Source: CAD feature listing. Evaluate the final solid. Frame: model axes, mm. A direction names the side the tool comes from. Give positions to 0.01 mm unless a question says otherwise; leave off trailing zeros. Order: outer loops, then holes, each group sorted by start corner. A loop starts at its lowest first (then second) coordinate and runs counter-clockwise, first axis right, second up.
from build123d import *

# Parameters (mm, degrees)
DODANIE_WYCI_GNI_CIE1_DEPTH = 1.9
DODANIE_WYCI_GNI_CIE3_DEPTH = 12.4
ESQUISSE4_R                 = 2.2
BOSS_EXTRU_2_DEPTH          = 2
ESQUISSE5_R                 = 1.1
ENL_V_MAT_EXTRU_2_DEPTH     = 29.971882921
ENL_V_MAT_EXTRU_4_REACH     = 38.806
ESQUISSE6_R                 = 1.1
ENL_V_START                 = -2.2
ESQUISSE7_R                 = 1.6
ESQUISSE7_R_2               = 1.1
ENL_V_MAT_EXTRU_5_DEPTH     = 2.2


with BuildPart() as part:
    # Szkic1 → Dodanie-wyciągnięcie1 (new body)
    with BuildSketch(Plane.XY):
        with BuildLine():
            Line((-12.9, 20), (12.9, 20))
            ThreePointArc((12.9, 20), (15.728427125, 18.828427125), (16.9, 16))
            Line((16.9, 16), (16.9, -16))
            ThreePointArc((16.9, -16), (15.728427125, -18.828427125), (12.9, -20))
            Line((12.9, -20), (-12.9, -20))
            ThreePointArc((-12.9, -20), (-15.728427125, -18.828427125), (-16.9, -16))
            Line((-16.9, -16), (-16.9, 16))
            ThreePointArc((-16.9, 16), (-15.728427125, 18.828427125), (-12.9, 20))
        make_face()
    extrude(amount=DODANIE_WYCI_GNI_CIE1_DEPTH)

    # Szkic3 → Dodanie-wyciągnięcie3 (add)
    with BuildSketch(Plane(origin=(0, 0, 0), x_dir=(-1, 0, 0), z_dir=(0, 0, -1))):
        Polygon((-9.4, -16.5), (-9.4, -11.5), (-11.4, -11.5), (-11.4, -18.5), (-2, -18.5), (-2, -11.5), (-6.5, -11.5), (-6.5, -16.5), align=None)
        Polygon((-9.4, 11.5), (-11.4, 11.5), (-11.4, 18.5), (-2, 18.5), (-2, 11.5), (-6.5, 11.5), (-6.5, 16.5), (-9.4, 16.5), align=None)
    extrude(amount=DODANIE_WYCI_GNI_CIE3_DEPTH)

    # Esquisse4 → Boss.-Extru.2 (add)
    with BuildSketch(Plane.ZY.offset(16.9)):
        with BuildLine():
            Line((-3.579120726, 8.391358342), (0, 5.442162864))
            Line((0, 5.442162864), (0, -5.442162864))
            Line((0, -5.442162864), (-8.920879274, 1.908641658))
            ThreePointArc((-8.920879274, 1.908641658), (-9.491358342, 7.820879274), (-3.579120726, 8.391358342))
        make_face()
        with Locations(Location((-6.25, 5.15, 0), (0, 0, 270))):
            Circle(ESQUISSE4_R, mode=Mode.SUBTRACT)
    extrude(amount=-BOSS_EXTRU_2_DEPTH)

    # Esquisse5 → Enlèv. mat.-Extru.2 (cut, through all)
    with BuildSketch(Plane(origin=(0, 0, 0), x_dir=(-1, 0, 0), z_dir=(0, 0, -1))):
        with Locations((6, 16)):
            Circle(ESQUISSE5_R)
        with Locations((6, -16)):
            Circle(ESQUISSE5_R)
    extrude(amount=-ENL_V_MAT_EXTRU_2_DEPTH, mode=Mode.SUBTRACT)

    # Enlèv. mat.-Extru.4: up to this face of the body (flat: up to its plane)
    enl_v_mat_extru_4_end = Plane(part.part.faces().sort_by_distance((2, 15, -6.2))[0])
    # Esquisse6 → Enlèv. mat.-Extru.4 (cut, up to the picked face)
    with BuildSketch(Plane(origin=(11.4, 0, 0), x_dir=(0, 0, -1), z_dir=(1, 0, 0)), mode=Mode.PRIVATE) as enl_v_mat_extru_4_sk1:
        with Locations((6.2, 13.9)):
            Circle(ESQUISSE6_R)
    enl_v_mat_extru_4_tool1 = split(extrude(enl_v_mat_extru_4_sk1.sketch, amount=-ENL_V_MAT_EXTRU_4_REACH, mode=Mode.PRIVATE), bisect_by=enl_v_mat_extru_4_end, keep=Keep.BOTH, mode=Mode.PRIVATE)
    # Esquisse6 → Enlèv. mat.-Extru.4 (cut, up to the picked face)
    with BuildSketch(Plane(origin=(11.4, 0, 0), x_dir=(0, 0, -1), z_dir=(1, 0, 0)), mode=Mode.PRIVATE) as enl_v_mat_extru_4_sk2:
        with Locations((6.2, -13.9)):
            Circle(ESQUISSE6_R)
    enl_v_mat_extru_4_tool2 = split(extrude(enl_v_mat_extru_4_sk2.sketch, amount=-ENL_V_MAT_EXTRU_4_REACH, mode=Mode.PRIVATE), bisect_by=enl_v_mat_extru_4_end, keep=Keep.BOTH, mode=Mode.PRIVATE)
    add(enl_v_mat_extru_4_tool1.solids().sort_by(Axis((11.4, 13.9, -6.2), (-1, 0, 0)))[0], mode=Mode.SUBTRACT)
    add(enl_v_mat_extru_4_tool2.solids().sort_by(Axis((11.4, -13.9, -6.2), (-1, 0, 0)))[0], mode=Mode.SUBTRACT)

    # Esquisse7 → Enlèv. mat.-Extru.5 (cut)
    # profile 1 of 4: a face of its own
    with BuildSketch(Plane.ZY.offset(-2).offset(ENL_V_START)):
        with Locations(Location((-6.2, 13.9, 0), (0, 0, 270))):
            Circle(ESQUISSE7_R)
        with Locations(Location((-6.2, 13.9, 0), (0, 0, 180))):
            Circle(ESQUISSE7_R_2, mode=Mode.SUBTRACT)
    # profile 2 of 4: a face of its own
    with BuildSketch(Plane.ZY.offset(-2).offset(ENL_V_START)):
        with Locations(Location((-6.2, 13.9, 0), (0, 0, 180))):
            Circle(ESQUISSE7_R_2)
    # profile 3 of 4: a face of its own
    with BuildSketch(Plane.ZY.offset(-2).offset(ENL_V_START)):
        with Locations(Location((-6.2, -13.9, 0), (0, 0, 270))):
            Circle(ESQUISSE7_R)
        with Locations(Location((-6.2, -13.9, 0), (0, 0, 270))):
            Circle(ESQUISSE7_R_2, mode=Mode.SUBTRACT)
    # profile 4 of 4: a face of its own
    with BuildSketch(Plane.ZY.offset(-2).offset(ENL_V_START)):
        with Locations(Location((-6.2, -13.9, 0), (0, 0, 270))):
            Circle(ESQUISSE7_R_2)
    extrude(amount=ENL_V_MAT_EXTRU_5_DEPTH, mode=Mode.SUBTRACT)


solid = part.part
1) First-contact query: pin 1 Ø4 at (x, y) = (5.5, -7.5) entering from -Z; pin 2 Ø5.5 at (y, z) = (13.5, -7) entering from +X; pin 3 Ø2.5 at (y, z) = (-13.9, -6.2) entering from -X; pin 4 Ø2 at (y, z) = (-13.9, -6.2) entering from -X. Flat tips, straight axial feed; report the tip coordinate or a pass-through.
Checks:
pin 1: stops at z = 0
pin 2: stops at x = 11.4
pin 3: stops at x = 4.2
pin 4: passes through
2) Section query A-A on x = -6. Output: boundary loops of the cut face in (y, z), and give its area (3 significant figures).
Checks:
outline: (-20, 0) - (-17.1, 0) - (-17.1, 1.9) - (-20, 1.9) - close; (-14.9, 0) - (14.9, 0) - (14.9, 1.9) - (-14.9, 1.9) - close; (17.1, 0) - (20, 0) - (20, 1.9) - (17.1, 1.9) - close
area: 67.6 mm2
3) Ray query, L1, parallel to Y at x = -6, z = 0.9; L2, parallel to X at y = 13, z = -4; L3, parallel to Y at x = 10.1, z = -6.2. Return the intervals inside material, ascending.
Checks:
L1: y = -20 to -17.1, -14.9 to 14.9, 17.1 to 20
L2: x = 2 to 6.5, 9.4 to 11.4
L3: y = -18.5 to -15, -12.8 to -11.5, 11.5 to 12.8, 15 to 18.5
4) Section query D-D on x = 10. Output: boundary loops of the cut face in (y, z).
Checks:
outline: (-20, 0) - (-18.5, 0) - (-18.5, -12.4) - (-11.5, -12.4) - (-11.5, 0) - (11.5, 0) - (11.5, -12.4) - (18.5, -12.4) - (18.5, 0) - (20, 0) - (20, 1.9) - (-20, 1.9) - close; hole circle Ø2.2 at (-13.9, -6.2); hole circle Ø2.2 at (13.9, -6.2)
5) Section query B-B on z = -1. Output: boundary loops of the cut face in (x, y), and give its area (3 significant figures).
Checks:
outline: (-16.9, -4.62) - (-14.9, -4.62) - (-14.9, 6.27) - (-16.9, 6.27) - close; (2, -18.5) - (11.4, -18.5) - (11.4, -11.5) - (9.4, -11.5) - (9.4, -16.5) - (6.5, -16.5) - (6.5, -11.5) - (2, -11.5) - close; (2, 11.5) - (6.5, 11.5) - (6.5, 16.5) - (9.4, 16.5) - (9.4, 11.5) - (11.4, 11.5) - (11.4, 18.5) - (2, 18.5) - close
area: 124 mm2
6) Pull-direction query (X, two-part tool) for faces 1 (the face through (15.759, -18.797, 0.937)), 2 (the face through (8, 16.5, -6)), 3 (the face through (2, 16, -6)); classes: +X half, -X half, draft (parallel to the pull), parting line (faces both ways), or undercut.
Checks:
face 1: +X half
face 2: undercut
face 3: -X half
7) Reachability of faces 4 (the face through (4.2, 15, -7)), 5 (the face through (6.5, 14, -4.7)), 6 (the face through (-14.9, 4, -4)) from +Z, -Z, +X, -X, +Y, -Y: full face, straight path, thin tool, end or side. Return the list, or none.
Checks:
face 4: -X
face 5: -Z
face 6: -Z, +X, +Y, -Y
8) Section query C-C on y = -13.9. Output: boundary loops of the cut face in (x, z), and give its area (3 significant figures).
Checks:
outline: (-16.9, 0) - (2, 0) - (2, -4.6) - (4.2, -4.6) - (4.2, -5.1) - (6.5, -5.1) - (6.5, 0) - (9.4, 0) - (9.4, -5.1) - (11.4, -5.1) - (11.4, 0) - (16.9, 0) - (16.9, 1.9) - (-16.9, 1.9) - close; (2, -12.4) - (6.5, -12.4) - (6.5, -7.3) - (4.2, -7.3) - (4.2, -7.8) - (2, -7.8) - close; (9.4, -12.4) - (11.4, -12.4) - (11.4, -7.3) - (9.4, -7.3) - close
area: 128 mm2
